Autodesk Inventor part; units mm, degrees
ref_plane "YZ Plane" through (0, 0, 0) normal (1, 0, 0) x (0, 1, 0)
ref_plane "XZ Plane" through (0, 0, 0) normal (0, 1, 0) x (-1, 0, 0)
ref_plane "XY Plane" through (0, 0, 0) normal (0, 0, 1) x (1, 0, 0)
sketch "Skizze1" plane through (0, 0, 0) normal (0, 1, 0) x (-1, 0, 0)
  circle A0 centre (0, 0) radius 19.1
  line L0 (-23.5, 23.5) -> (23.5, 23.5) construction
  line L1 (23.5, 23.5) -> (23.5, -23.5) construction
  line L2 (23.5, -23.5) -> (-23.5, -23.5) construction
  line L3 (-23.5, -23.5) -> (-23.5, 23.5) construction
  line L4 (-23.5, 23.5) -> (23.5, -23.5) construction
  line L5 (23.5, 23.5) -> (-23.5, -23.5) construction
  circle A1 centre (23.5, -23.5) radius 2.2
  circle A2 centre (23.5, 23.5) radius 2.2
  circle A3 centre (-23.5, 23.5) radius 2.2
  circle A4 centre (-23.5, -23.5) radius 2.2
  line L6 (-40, 40) -> (40, 40)
  line L7 (40, 40) -> (40, -40)
  line L8 (40, -40) -> (-40, -40)
  line L9 (-40, -40) -> (-40, 40)
  line L10 (-40, 40) -> (40, -40) construction
  line L11 (40, 40) -> (-40, -40) construction
  line L12 (-32.75, 23.5) -> (32.75, 23.5) construction
  line L13 (32.75, 23.5) -> (32.75, -23.5) construction
  line L14 (32.75, -23.5) -> (-32.75, -23.5) construction
  line L15 (-32.75, -23.5) -> (-32.75, 23.5) construction
  line L16 (-32.75, 23.5) -> (32.75, -23.5) construction
  line L17 (32.75, 23.5) -> (-32.75, -23.5) construction
  line L18 (32.75, -18.5) -> (32.75, -28.5) construction
  line L19 (31.05, -18.5) -> (31.05, -28.5)
  line L20 (34.45, -28.5) -> (34.45, -18.5)
  arc A5 (34.45, -18.5) -> (31.05, -18.5) centre (32.75, -18.5) ccw
  arc A6 (31.05, -28.5) -> (34.45, -28.5) centre (32.75, -28.5) ccw
  line L21 (32.75, 28.5) -> (32.75, 18.5) construction
  line L22 (31.05, 28.5) -> (31.05, 18.5)
  line L23 (34.45, 18.5) -> (34.45, 28.5)
  arc A7 (34.45, 28.5) -> (31.05, 28.5) centre (32.75, 28.5) ccw
  arc A8 (31.05, 18.5) -> (34.45, 18.5) centre (32.75, 18.5) ccw
  line L24 (-32.75, 28.5) -> (-32.75, 18.5) construction
  line L25 (-34.45, 28.5) -> (-34.45, 18.5)
  line L26 (-31.05, 18.5) -> (-31.05, 28.5)
  arc A9 (-31.05, 28.5) -> (-34.45, 28.5) centre (-32.75, 28.5) ccw
  arc A10 (-34.45, 18.5) -> (-31.05, 18.5) centre (-32.75, 18.5) ccw
  line L27 (-32.75, -18.5) -> (-32.75, -28.5) construction
  line L28 (-34.45, -18.5) -> (-34.45, -28.5)
  line L29 (-31.05, -28.5) -> (-31.05, -18.5)
  arc A11 (-31.05, -18.5) -> (-34.45, -18.5) centre (-32.75, -18.5) ccw
  arc A12 (-34.45, -28.5) -> (-31.05, -28.5) centre (-32.75, -28.5) ccw
  line L30 (-30, 30) -> (30, 30)
  line L31 (30, 30) -> (30, -30)
  line L32 (30, -30) -> (-30, -30)
  line L33 (-30, -30) -> (-30, 30)
  line L34 (-30, 30) -> (30, -30) construction
  line L35 (30, 30) -> (-30, -30) construction
  dimension "d31" = 38.2
  dimension "d32" = 47
  dimension "d33" = 47
  dimension "d34" = 4.4
  dimension "d35" = 4.4
  dimension "d36" = 4.4
  dimension "d37" = 4.4
  dimension "d38" = 80
  dimension "d39" = 80
  dimension "d40" = 65.5
  dimension "d41" = 47
  dimension "d42" = 5
  dimension "d43" = 3.4
  dimension "d44" = 5
  dimension "d45" = 3.4
  dimension "d46" = 5
  dimension "d47" = 3.4
  dimension "d48" = 5
  dimension "d49" = 3.4
  dimension "d50" = 60
  dimension "d51" = 60
extrude "Extrusion1" add sketch "Skizze1" against normal blind 10 contours L6 L7 L8 L9
extrude "Extrusion2" add sketch "Skizze1" against normal blind 5 contours L30 L31 L32 L33
fillet "Rundung1" radius 2 8 edges at (-40, -5, 40) (40, -5, -40) (-40, -5, -40) (40, -5, 40) (30, -7.5, 30) (-30, -7.5, -30) (30, -7.5, -30) (-30, -7.5, 30)
chamfer "Fase1" distance 0.2 angle 45 33 edges at (25.7, -5, 23.5) (30, -10, 0) (0, -10, -30) (-30, -10, 0) (0, -10, 30) (32.75, -10, 16.8) (31.05, -10, 23.5) (32.75, -10, 30.2) (34.45, -10, 23.5) (19.1, -5, 0) (25.7, -5, -23.5) (-21.3, -5, -23.5) (-21.3, -5, 23.5) (-32.75, -10, 16.8) (-34.45, -10, 23.5) (-32.75, -10, 30.2) (-31.05, -10, 23.5) (-32.75, -10, -16.8) (-31.05, -10, -23.5) (-32.75, -10, -30.2) (-34.45, -10, -23.5) (0, -10, -40) (39.4142, -10, -39.4142) (40, -10, 0) (39.4142, -10, 39.4142) (0, -10, 40) (-39.4142, -10, 39.4142) (-40, -10, 0) (-39.4142, -10, -39.4142) (32.75, -10, -16.8) (34.45, -10, -23.5) (32.75, -10, -30.2) (31.05, -10, -23.5)
thread "Gewinde1"
thread "Gewinde2"
thread "Gewinde3"
thread "Gewinde4"
properties part number "Z-Motoraufnahme" material "Aluminium 6061"
The listing builds one solid part. Answer for the finished solid, in the listing's coordinates (mm). A direction names the side the tool comes from. Round coordinates to 2 decimals unless told otherwise and drop trailing zeros. Write each loop counter-clockwise with the first axis right and the second up, starting at its lowest first coordinate (ties: lowest second). Pieces come first, ordered by that corner, then holes. Notation, with made-up numbers: (6.5, -9) - (43.5, -9) arc R13 ccw to (43.5, -3) - close; hole circle Ø8 at (2.25, -22.75). An arc over 180 degrees is marked (long way). Use one line per item in the form item = value. Start each with the question number.
Item 1: A flat-ended cylindrical pin translates along its axis: pin 1 Ø1.5 at (x, z) = (-26.5, 0) entering from -Y. Find the tip coordinate at first contact, or state that the pin passes through.
Item 2: Find the intervals of material crossed by line 1 (X direction, y = -7, z = -19.5); line 2 (Z direction, x = -23.5, y = -1.05); line 3 (Z direction, x = -32.5, y = -4.25), in increasing order. Write a range as [from, to].
Item 3: A cutting plane is placed at A-A (x = 32.75). Write down the section's boundary in (y, z).
Item 4: A cutting plane is placed at D-D (x = -23.5). Write down the section's boundary in (y, z), plus the area to 3 significant figures.
Item 5: A cutting plane is placed at B-B (z = 0). Write down the section's boundary in (x, y), plus the area to 3 significant figures.
Item 6: A tool of negligible diameter and unlimited length cuts with its end or side. For faces 1 (the cylindrical face through (-32.8, -4.8, 30.2)), 2 (the flat face through (1, -5, 40)), 3 (the cylindrical face through (-29.43, -7.43, -29.4)), from which of +Z, -Z, +X, -X, +Y, -Y can it reach the whole face along a straight path? Write none if from no direction.
Item 7: A cutting plane is placed at C-C (y = -1.75). Give the number of separate pieces and of enclosed holes in the cut face, plus the area to 3 significant figures.
Item 8: Determine the mould class of faces 4 (the cylindrical face through (32.7, -4.8, 30.2)), 5 (the cylindrical face through (39.4, -4.97, -39.43)), 6 (the flat face through (-40, -5, 1)) for opening direction X: +X half, -X half, draft (parallel to the pull), parting line (faces both ways), or undercut.
The answers:
q1.pin_1 = -5
q2.line_1 = [-40, -34.45], [-31.05, -30], [30, 31.05], [34.45, 40]
q2.line_2 = [-40, -25.7], [-21.3, 21.3], [25.7, 40]
q2.line_3 = [-40, -30.18], [-16.82, 16.82], [30.18, 40]
q3.outline = (-10, -39.8) - (-9.8, -40) - (0, -40) - (0, -30.2) - (-9.8, -30.2) - (-10, -30.4) - close; (-10, -16.6) - (-9.8, -16.8) - (0, -16.8) - (0, 16.8) - (-9.8, 16.8) - (-10, 16.6) - close; (-10, 30.4) - (-9.8, 30.2) - (0, 30.2) - (0, 40) - (-9.8, 40) - (-10, 39.8) - close
q4.outline = (-10, -39.8) - (-9.8, -40) - (0, -40) - (0, -25.7) - (-4.8, -25.7) - (-5, -25.9) - (-5, -30) - (-9.8, -30) - (-10, -30.2) - close; (-10, 30.2) - (-9.8, 30) - (-5, 30) - (-5, 25.9) - (-4.8, 25.7) - (0, 25.7) - (0, 40) - (-9.8, 40) - (-10, 39.8) - close; (-5, -21.1) - (-4.8, -21.3) - (0, -21.3) - (0, 21.3) - (-4.8, 21.3) - (-5, 21.1) - close
q4.area = 456 mm^2
q5.outline = (-40, -9.8) - (-39.8, -10) - (-30.2, -10) - (-30, -9.8) - (-30, -5) - (-19.3, -5) - (-19.1, -4.8) - (-19.1, 0) - (-40, 0) - close; (19.1, -4.8) - (19.3, -5) - (30, -5) - (30, -9.8) - (30.2, -10) - (39.8, -10) - (40, -9.8) - (40, 0) - (19.1, 0) - close
q5.area = 309 mm^2
q6.face_1 = +Y, -Y
q6.face_2 = +Z, +X, -X, +Y, -Y
q6.face_3 = -Y
q7.separate_pieces = 1
q7.enclosed_holes = 9
q7.area = 5,020 mm^2
q8.face_4 = undercut
q8.face_5 = +X half
q8.face_6 = -X half
